Source: CAD feature listing. Evaluate the final solid. Frame: model axes, mm. A direction names the side the tool comes from. Give positions to 0.01 mm unless a question says otherwise; leave off trailing zeros. Loops run counter-clockwise (first coordinate to the right, second up) from the corner with the lowest first, then second, coordinate; pieces in that order, holes last.
```python
from build123d import *

# Parameters (mm, degrees)
SKETCH_1_W                      = 106
SKETCH_1_H                      = 105
EXTRUDE_1_DEPTH                 = 40
CUT_EXTRUDE_1_DEPTH             = 125.233650836
CUT_EXTRUDE_1_DEPTH_BACK        = 125.233650836
SKETCH_3_W                      = 100
SKETCH_3_H                      = 99
CUT_EXTRUDE_3_DEPTH             = 1
CUT_EXTRUDE_3_DEPTH_BACK        = 3
SKETCH_7_R                      = 2.5
SKETCH_7_R_2                    = 1.6
CUT_EXTRUDE_4_REACH             = 126.234
SKETCH_6_W                      = 13
SKETCH_6_H                      = 25
CUT_EXTRUDE_4_DIRECTION_2_DEPTH = 125.233650836
CUT_EXTRUDE_5_DEPTH             = 155.470061824
CUT_EXTRUDE_5_DEPTH_BACK        = 155.470061824
SKETCH_10_W                     = 13
SKETCH_10_H                     = 25
CUT_EXTRUDE_6_DEPTH             = 155.470061824
CUT_EXTRUDE_6_DEPTH_BACK        = 155.470061824


with BuildPart() as part:
    # 草图1 → 凸台-拉伸1 (new body)
    with BuildSketch(Plane.XY):
        with Locations((0, 52.5)):
            Rectangle(SKETCH_1_W, SKETCH_1_H)
    extrude(amount=EXTRUDE_1_DEPTH)

    # 草图3 → 切除-拉伸1 (cut, two sides: drawn at the far end of the back side and taken through both)
    with BuildSketch(Plane(origin=(0, 0, 0), x_dir=(-1, 0, 0), z_dir=(0, 0, -1)).offset(-CUT_EXTRUDE_1_DEPTH_BACK)):
        with Locations((0, 52.5)):
            Rectangle(SKETCH_3_W, SKETCH_3_H)
    extrude(amount=CUT_EXTRUDE_1_DEPTH + CUT_EXTRUDE_1_DEPTH_BACK, mode=Mode.SUBTRACT)

    # 草图7 → 切除-拉伸3 (cut, two sides: drawn at the far end of the back side and taken through both)
    with BuildSketch(Plane.XZ.offset(-CUT_EXTRUDE_3_DEPTH_BACK)):
        with Locations(Location((0, 20, 0), (0, 0, 180))):
            Circle(SKETCH_7_R)
        with Locations(Location((5, 25, 0), (0, 0, 180))):
            Circle(SKETCH_7_R_2)
        with Locations(Location((5, 15, 0), (0, 0, 180))):
            Circle(SKETCH_7_R_2)
        with Locations(Location((-5, 15, 0), (0, 0, 180))):
            Circle(SKETCH_7_R_2)
        with Locations(Location((-5, 25, 0), (0, 0, 180))):
            Circle(SKETCH_7_R_2)
        with Locations(Location((15, 25, 0), (0, 0, 180))):
            Circle(SKETCH_7_R_2)
        with Locations(Location((-15, 25, 0), (0, 0, 180))):
            Circle(SKETCH_7_R_2)
        with Locations(Location((15, 15, 0), (0, 0, 180))):
            Circle(SKETCH_7_R_2)
        with Locations(Location((-15, 15, 0), (0, 0, 180))):
            Circle(SKETCH_7_R_2)
    extrude(amount=CUT_EXTRUDE_3_DEPTH + CUT_EXTRUDE_3_DEPTH_BACK, mode=Mode.SUBTRACT)

    # 草图6 → 切除-拉伸4 (cut, up to next)
    with BuildSketch(Plane(origin=(0, 105, 0), x_dir=(1, 0, 0), z_dir=(0, 1, 0)), mode=Mode.PRIVATE) as cut_extrude_4_sk1:
        with Locations((0, -20)):
            Rectangle(SKETCH_6_W, SKETCH_6_H)
    cut_extrude_4_tool1 = extrude(cut_extrude_4_sk1.sketch, amount=-CUT_EXTRUDE_4_REACH, mode=Mode.PRIVATE) & part.part
    add(cut_extrude_4_tool1.solids().sort_by_distance((0, 105, 20))[0], mode=Mode.SUBTRACT)

    # 草图6 → 切除-拉伸4 direction 2 (cut)
    with BuildSketch(Plane(origin=(0, 105, 0), x_dir=(1, 0, 0), z_dir=(0, 1, 0))):
        with Locations((0, -20)):
            Rectangle(SKETCH_6_W, SKETCH_6_H)
    extrude(amount=CUT_EXTRUDE_4_DIRECTION_2_DEPTH, mode=Mode.SUBTRACT)

    # 草图10 → 切除-拉伸5 (cut, two sides: drawn at the far end of the back side and taken through both)
    with BuildSketch(Plane.ZY.offset(53).offset(-CUT_EXTRUDE_5_DEPTH_BACK)):
        with Locations((20, 87.306952357)):
            Rectangle(SKETCH_10_W, SKETCH_10_H)
    extrude(amount=CUT_EXTRUDE_5_DEPTH + CUT_EXTRUDE_5_DEPTH_BACK, mode=Mode.SUBTRACT)

    # 草图12 → 切除-拉伸6 (cut, two sides: drawn at the far end of the back side and taken through both)
    with BuildSketch(Plane(origin=(53, 0, 0), x_dir=(0, 0, -1), z_dir=(1, 0, 0)).offset(-CUT_EXTRUDE_6_DEPTH_BACK)):
        with BuildLine():
            Line((-30.108588081, 25.649961527), (-30.108588081, 47.398469004))
            ThreePointArc((-30.108588081, 47.398469004), (-20, 57.507057086), (-9.891411919, 47.398469004))
            Line((-9.891411919, 47.398469004), (-9.891411919, 25.649961527))
            ThreePointArc((-9.891411919, 25.649961527), (-20, 15.541373446), (-30.108588081, 25.649961527))
        make_face()
    extrude(amount=CUT_EXTRUDE_6_DEPTH + CUT_EXTRUDE_6_DEPTH_BACK, mode=Mode.SUBTRACT)


solid = part.part
```
(1) Mould query, pull axis X, two halves, no side actions, for faces 1 (the cylindrical face through (5.208, 1.521, 23.414)), 2 (the flat face through (53, 63, 20)), 3 (the flat face through (51, 36, 30.109)). Classes: pulls with the +X half, pulls with the -X half, needs draft (parallel to the pull), parting line crosses it, or undercut.
A:
face 1: undercut
face 2: pulls with the +X half
face 3: needs draft
(2) First-contact query: pin 1 (3 mm diameter, centred on x = 15, z = 25, fed in from -Y). Flat tip, straight axial feed; report the tip coordinate or a pass-through.
A:
pin 1: stops at y = 102
(3) Ray query, line 1 along X through (y, z) = (1, 15); line 2 along Z through (x, y) = (15, 2); line 3 along Y through (x, z) = (22, 24.5). Return the intervals inside material, ascending.
A:
line 1: x = -53 to -16.6, -13.4 to -6.6, -3.4 to 3.4, 6.6 to 13.4, 16.6 to 53
line 2: z = 0 to 13.4, 16.6 to 23.4, 26.6 to 40
line 3: y = 0 to 3, 102 to 105
(4) Section B-B, the plane y = 30. Return the cut outline in (x, z), then the cut area to 3 significant figures.
A:
outline: (-53, 0) - (-50, 0) - (-50, 9.89) - (-53, 9.89) - close; (-53, 30.11) - (-50, 30.11) - (-50, 40) - (-53, 40) - close; (50, 0) - (53, 0) - (53, 9.89) - (50, 9.89) - close; (50, 30.11) - (53, 30.11) - (53, 40) - (50, 40) - close
area: 119 mm2
(5) Section D-D, the plane z = 35.5. Return the cut outline in (x, y), then the cut area to 3 significant figures.
A:
outline: (-53, 0) - (53, 0) - (53, 105) - (-53, 105) - close; hole (-50, 3) - (50, 3) - (50, 102) - (-50, 102) - close
area: 1,230 mm2
(6) Section C-C, the plane x = 0. Return the cut outline in (y, z).
A:
outline: (0, 0) - (3, 0) - (3, 17.5) - (0, 17.5) - close; (0, 22.5) - (3, 22.5) - (3, 40) - (0, 40) - close; (102, 0) - (105, 0) - (105, 7.5) - (102, 7.5) - close; (102, 32.5) - (105, 32.5) - (105, 40) - (102, 40) - close
(7) Reachability of faces 4 (the cylindrical face through (51.479, 57.505, 20.222)), 5 (the cylindrical face through (16.18, 1.52, 13.92)), 6 (the flat face through (12, 102, 20)), 7 (the flat face through (-6.5, 104, 20)) from +Z, -Z, +X, -X, +Y, -Y: full face, straight path, thin tool, end or side. Return the list, or none.
A:
face 4: +X, -X
face 5: -Y
face 6: +Z, -Z
face 7: +Y
(8) Section A-A, the plane x = 37. Return the cut outline in (y, z).
A:
outline: (0, 0) - (3, 0) - (3, 40) - (0, 40) - close; (102, 0) - (105, 0) - (105, 40) - (102, 40) - close
